For this review, take the finished solid that the model builds, in its own axes (mm). Face numbers are marked on the shaded views. A direction names the side the tool comes from. Round coordinates to 2 decimals unless told otherwise and drop trailing zeros. Loops run counter-clockwise (first coordinate to the right, second up) from the corner with the lowest first, then second, coordinate; pieces in that order, holes last.
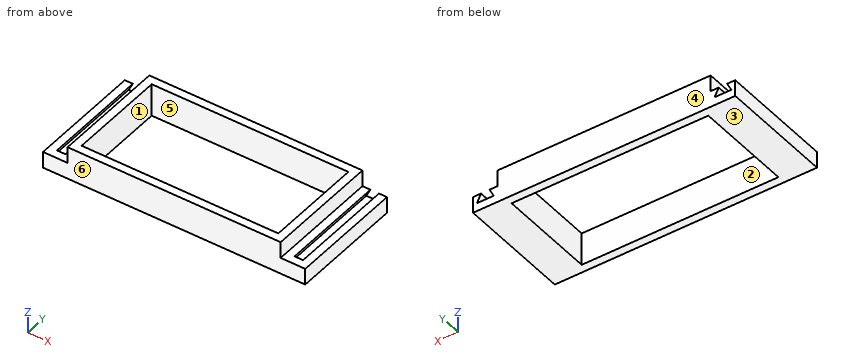
Autodesk Inventor part; units mm, degrees
ref_plane "YZ Plane" through (0, 0, 0) normal (1, 0, 0) x (0, 1, 0)
ref_plane "XZ Plane" through (0, 0, 0) normal (0, 1, 0) x (-1, 0, 0)
ref_plane "XY Plane" through (0, 0, 0) normal (0, 0, 1) x (1, 0, 0)
sketch "Sketch2" plane through (0, 0, 0) normal (0, 0, 1) x (1, 0, 0)
  line L0 (0, 0) -> (203.2, 0)
  line L1 (203.2, 0) -> (203.2, 88.9)
  line L2 (203.2, 88.9) -> (0, 88.9)
  line L3 (0, 88.9) -> (0, 0)
  dimension "d6" = 203.2
  dimension "d7" = 88.9
extrude "Extrusion2" add sketch "Sketch2" along normal blind 12.7
sketch "Sketch3" plane through (0, 0, 12.7) normal (0, 0, 1) x (1, 0, 0)
  line L0 (0, 0) -> (203.2, 0)
  line L1 (203.2, 0) -> (203.2, 88.9)
  line L2 (203.2, 88.9) -> (0, 88.9)
  line L3 (0, 88.9) -> (0, 0)
  line L4 (203.2, 88.9) -> (0, 88.9) construction
  line L5 (0, 0) -> (203.2, 0) construction
  line L6 (0, 88.9) -> (203.2, 0) construction
  line L7 (203.2, 0) -> (203.2, 88.9) construction
  line L8 (203.2, 88.9) -> (0, 0) construction
  line L9 (25.4, 6.35) -> (177.8, 6.35)
  line L10 (177.8, 6.35) -> (177.8, 82.55)
  line L11 (177.8, 82.55) -> (25.4, 82.55)
  line L12 (25.4, 82.55) -> (25.4, 6.35)
  line L13 (25.4, 6.35) -> (177.8, 82.55) construction
  line L14 (177.8, 6.35) -> (25.4, 82.55) construction
  line L15 (19.05, 88.9) -> (184.15, 88.9)
  line L16 (184.15, 88.9) -> (184.15, 0)
  line L17 (184.15, 0) -> (19.05, 0)
  line L18 (19.05, 0) -> (19.05, 88.9)
  point P0 (101.6, 44.45)
  dimension "d10" = 152.4
  dimension "d11" = 76.2
  dimension "d12" = 6.35
extrude "Extrusion3" add sketch "Sketch3" along normal blind 12.7 contours L18 L2 L16 L0
sketch "Sketch5" plane through (0, 88.9, 0) normal (0, 1, 0) x (1, 0, 0)
  line L0 (203.2, 0) -> (0, 0)
  line L1 (0, 0) -> (0, -12.7)
  line L2 (19.05, -12.7) -> (0, -12.7)
  line L3 (19.05, -12.7) -> (19.05, -25.4)
  line L4 (184.15, -25.4) -> (19.05, -25.4)
  line L5 (184.15, -12.7) -> (184.15, -25.4)
  line L6 (203.2, -12.7) -> (184.15, -12.7)
  line L7 (203.2, 0) -> (203.2, -12.7)
  line L8 (0, 0) -> (203.2, 0) construction
  line L9 (0, -12.7) -> (19.05, -12.7)
  line L10 (19.05, -12.7) -> (19.05, 0) construction
  line L11 (19.05, 0) -> (0, 0) construction
  line L12 (0, 0) -> (0, -12.7) construction
  line L13 (19.05, -12.7) -> (0, -12.7) construction
  line L14 (9.525, -12.7) -> (9.525, -6.3424) construction
  line L15 (9.525, -12.7) -> (12.827, -12.7) construction
  line L16 (9.525, -12.7) -> (6.223, -12.7)
  line L17 (9.525, -6.3424) -> (16.002, -6.3424)
  line L18 (9.525, -6.3424) -> (3.048, -6.3424)
  line L19 (3.048, -6.3424) -> (6.223, -12.7)
  line L20 (6.223, -12.7) -> (-12.7, -12.7)
  line L21 (193.6826, 0) -> (193.675, -12.7) construction
  line L22 (193.675, -12.7) -> (196.977, -12.7)
  line L23 (184.15, -12.7) -> (203.2, -12.7)
  line L24 (193.675, -12.7) -> (190.373, -12.7)
  line L25 (193.675, -12.7) -> (193.6788, -6.35) construction
  line L26 (9.525, -12.7) -> (9.525, -6.35) construction
  line L27 (16.002, -6.3424) -> (12.827, -12.7)
  line L28 (196.977, -12.7) -> (190.373, -12.7)
  line L29 (3.048, -6.3424) -> (6.223, -12.7)
  line L30 (6.223, -12.7) -> (12.827, -12.7)
  line L31 (12.827, -12.7) -> (16.002, -6.3424)
  line L32 (16.002, -6.3424) -> (3.048, -6.3424)
  line L33 (193.6788, -6.35) -> (187.2018, -6.35)
  line L34 (193.6788, -6.35) -> (200.1558, -6.35)
  line L35 (187.2018, -6.35) -> (190.373, -12.7)
  line L36 (200.1558, -6.35) -> (196.977, -12.7)
  dimension "d15" = 3.302
  dimension "d16" = 3.302
  dimension "d17" = 6.477
  dimension "d18" = 6.477
  dimension "d19" = 3.302
  dimension "d20" = 3.302
  dimension "d25" = 6.35
  dimension "d26" = 6.35
  dimension "d31" = 6.477
  dimension "d32" = 6.477
extrude "Extrusion5" cut sketch "Sketch5" against normal blind 82.55 contours L6 L35 L33 L34 L36 | L19 L18 L17 L27 L2
sketch "Sketch6" plane through (0, 0, 12.7) normal (0, 0, 1) x (1, 0, 0)
  line L0 (25.4, 82.55) -> (25.4, 6.35)
  line L1 (25.4, 6.35) -> (177.8, 6.35)
  line L2 (25.4, 82.55) -> (177.8, 82.55)
  line L3 (177.8, 82.55) -> (177.8, 6.35)
  line L4 (177.8, 6.35) -> (25.4, 6.35)
  line L5 (25.4, 6.35) -> (25.4, 82.55)
  point P0 (0, 0)
extrude "Extrusion6" cut sketch "Sketch6" against normal blind 82.55
properties part number "doveTailSide"
(1) The part is to be moulded in two halves that separate along Y. For the marked faces 1, 2, 3 and 4, say which applies: pulls with the +Y half, pulls with the -Y half, needs draft (parallel to the pull), parting line crosses it, or undercut.
(2) Add section B-B (y = 12). Give the boundary of the cut face in (x, z).
(3) Add section A-A (x = 45.5). Give the boundary of the cut face in (y, z).
(4) For the marked faces 5 and 6, list the 3-axis set-ups (+Z, -Z, +X, -X, +Y, -Y) from which the entire face can be reached by the end or side of a thin tool; tool diameter is ignored.
(5) For L1, parallel to X at y = 67, z = 15.75; L2, parallel to Y at x = 29, z = 8.5; L3, parallel to X at y = 45, z = 2.25, list the stretches that pass through material, from the lowest coordinate up.
(6) Add section C-C (z = 19.75). Give the boundary of the cut face in (x, y).
(7) Insertion check: pin 1 Ø6 at (x, y) = (30, 46.5) entering from +Z; pin 2 Ø4 at (y, z) = (34, 17) entering from +X; pin 3 Ø6.5 at (y, z) = (24.5, 19) entering from -X; pin 4 Ø5 at (x, z) = (194, 8) entering from +Y. Each pin has a flat end and moves straight along its axis. Give the tip position at first contact, or say it passes through.
Outcome:
1. face 1: undercut
1. face 2: undercut
1. face 3: needs draft
1. face 4: pulls with the +Y half
2. outline: (0, 0) - (25.4, 0) - (25.4, 25.4) - (19.05, 25.4) - (19.05, 12.7) - (12.83, 12.7) - (16, 6.34) - (3.05, 6.34) - (6.22, 12.7) - (0, 12.7) - close; (177.8, 0) - (203.2, 0) - (203.2, 12.7) - (196.98, 12.7) - (200.16, 6.35) - (187.2, 6.35) - (190.37, 12.7) - (184.15, 12.7) - (184.15, 25.4) - (177.8, 25.4) - close
3. outline: (0, 0) - (6.35, 0) - (6.35, 25.4) - (0, 25.4) - close; (82.55, 0) - (88.9, 0) - (88.9, 25.4) - (82.55, 25.4) - close
4. face 5: +Z, -Z
4. face 6: +Z, -Z, +X, -X, -Y
5. L1: x = 19.05 to 25.4, 177.8 to 184.15
5. L2: y = 0 to 6.35, 82.55 to 88.9
5. L3: x = 0 to 25.4, 177.8 to 203.2
6. outline: (19.05, 0) - (184.15, 0) - (184.15, 88.9) - (19.05, 88.9) - close; hole (25.4, 6.35) - (177.8, 6.35) - (177.8, 82.55) - (25.4, 82.55) - close
7. pin 1: passes through
7. pin 2: stops at x = 184.15
7. pin 3: stops at x = 19.05
7. pin 4: stops at y = 88.9
